The listing builds one solid part. Answer for the finished solid, in the listing's coordinates (mm). Face numbers are marked on the shaded views. A direction names the side the tool comes from. Give positions to 0.01 mm unless a question says otherwise; leave off trailing zeros. Order: outer loops, then holes, each group sorted by start corner. A loop starts at its lowest first (then second) coordinate and runs counter-clockwise, first axis right, second up.
```python
from build123d import *

# Parameters (mm, degrees)
F0_W     = 36
F0_H     = 12
F0_R     = 1.3
F1_DEPTH = 5
F0_W_2   = 12
F0_H_2   = 5
F0_H_3   = 1
F0_H_4   = 2
F2_DEPTH = 2
F3_DEPTH = 8
F4_R     = 2


with BuildPart() as f1:
    # F0 (on Top) → F1 (new body)
    with BuildSketch(Plane.XY):
        with Locations((0, -11)):
            Rectangle(F0_W, F0_H)
        with Locations((-15.25, -14.5)):
            Circle(F0_R, mode=Mode.SUBTRACT)
        with Locations((15.25, -14.5)):
            Circle(F0_R, mode=Mode.SUBTRACT)
    extrude(amount=F1_DEPTH)



with BuildPart() as f1b:
    # F0 (on Top) → F1, piece 2 (new body)
    with BuildSketch(Plane.XY):
        with Locations((-12, 14.5)):
            Rectangle(F0_W_2, F0_H_2)
        with Locations((-15.25, 14.5)):
            Circle(F0_R, mode=Mode.SUBTRACT)
    extrude(amount=F1_DEPTH)


with BuildPart() as f1c:
    # F0 (on Top) → F1, piece 3 (new body)
    with BuildSketch(Plane.XY):
        with Locations((12, 14.5)):
            Rectangle(F0_W_2, F0_H_2)
        with Locations((15.25, 14.5)):
            Circle(F0_R, mode=Mode.SUBTRACT)
    extrude(amount=F1_DEPTH)


with BuildPart() as f1_1:
    add(f1.part)

    add(f1b.part)  # F2 merges F1b

    add(f1c.part)  # F2 merges F1c
    # F0 (on Top) → F2 (join)
    with BuildSketch(Plane.XY):
        Polygon((-6, 12), (-18, 12), (-18, -5), (18, -5), (18, 12), (6, 12), align=None)
        with Locations((0, 14.5)):
            Rectangle(F0_W_2, F0_H_2)
        Polygon((-18, 12), (-18, 17), (-6, 17), (-6, 18), (-19, 18), (-19, -18), (19, -18), (19, 18), (6, 18), (6, 17), (18, 17), (18, 12), (18, -5), (18, -17), (-18, -17), (-18, -5), align=None)
        with Locations((0, 17.5)):
            Rectangle(F0_W_2, F0_H_3)
        with Locations((0, 19)):
            Rectangle(F0_W_2, F0_H_4)
    extrude(amount=F2_DEPTH)

    # F0 (on Top) → F3 (join)
    with BuildSketch(Plane.XY):
        with Locations((-15.25, 14.5)):
            Circle(F0_R)
        with Locations((15.25, 14.5)):
            Circle(F0_R)
        with Locations((15.25, -14.5)):
            Circle(F0_R)
        with Locations((-15.25, -14.5)):
            Circle(F0_R)
        Polygon((-19, 18), (-6, 18), (-6, 20), (-21, 20), (-21, -20), (21, -20), (21, 20), (6, 20), (6, 18), (19, 18), (19, -18), (-19, -18), align=None)
    extrude(amount=F3_DEPTH)

    # F4
    f4_edges = [f1_1.edges().sort_by_distance(p)[0] for p in [
        (-21, -20, 4),
        (21, -20, 4),
        (21, 20, 4),
        (-21, 20, 4),
    ]]
    fillet(f4_edges, radius=F4_R)


solid = f1_1.part
```
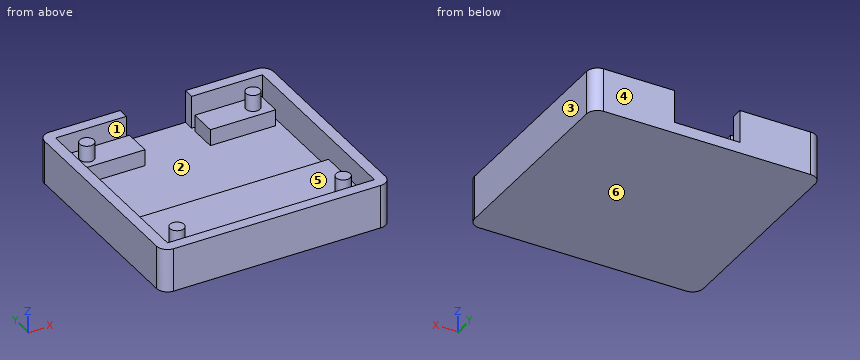
1) For a pull along X with two mould halves and no side action, classify the marked faces 1, 2, 3 and 4 as +X half, -X half, draft (parallel to the pull), parting line (faces both ways), or undercut.
Geometry says:
face 1: undercut
face 2: undercut
face 3: +X half
face 4: draft
2) Find section C-C (x = -3.5). Write down the section's boundary in (y, z).
Geometry says:
outline: (-20, 0) - (20, 0) - (20, 2) - (-5, 2) - (-5, 5) - (-17, 5) - (-17, 2) - (-18, 2) - (-18, 8) - (-20, 8) - close
3) Straight lines are drawn through the part: probe 1 along Y at (x, z) = (15, 4); probe 2 along X at (y, z) = (6.5, 3.5); probe 3 along X at (y, z) = (-10, 4.25). For each, find the intervals that lie inside material, in ascending order.
Geometry says:
probe 1: y = -20 to -18, -17 to -5, 12 to 17, 18 to 20
probe 2: x = -21 to -19, 19 to 21
probe 3: x = -21 to -19, -18 to 18, 19 to 21
4) Find section A-A (z = 3.25). Write down the section's boundary in (x, y), then the cut area to 3 significant figures.
Geometry says:
outline: (-21, -18) arc R2 ccw to (-19, -20) - (19, -20) arc R2 ccw to (21, -18) - (21, 18) arc R2 ccw to (19, 20) - (6, 20) - (6, 18) - (19, 18) - (19, -18) - (-19, -18) - (-19, 18) - (-6, 18) - (-6, 20) - (-19, 20) arc R2 ccw to (-21, 18) - close; (-18, -17) - (18, -17) - (18, -5) - (-18, -5) - close; (-18, 12) - (-6, 12) - (-6, 17) - (-18, 17) - close; (6, 12) - (18, 12) - (18, 17) - (6, 17) - close
area: 837 mm2
5) Find section B-B (y = 16.5). Write down the section's boundary in (x, z).
Geometry says:
outline: (-21, 0) - (21, 0) - (21, 8) - (19, 8) - (19, 2) - (18, 2) - (18, 5) - (6, 5) - (6, 2) - (-6, 2) - (-6, 5) - (-18, 5) - (-18, 2) - (-19, 2) - (-19, 8) - (-21, 8) - close
6) Find section D-D (z = 7.5). Write down the section's boundary in (x, y).
Geometry says:
outline: (-21, -18) arc R2 ccw to (-19, -20) - (19, -20) arc R2 ccw to (21, -18) - (21, 18) arc R2 ccw to (19, 20) - (6, 20) - (6, 18) - (19, 18) - (19, -18) - (-19, -18) - (-19, 18) - (-6, 18) - (-6, 20) - (-19, 20) arc R2 ccw to (-21, 18) - close; circle Ø2.6 at (-15.25, -14.5); circle Ø2.6 at (-15.25, 14.5); circle Ø2.6 at (15.25, -14.5); circle Ø2.6 at (15.25, 14.5)
7) A tool of negligible diameter and unlimited length cuts with its end or side. For the marked faces 5 and 6, from which of +Z, -Z, +X, -X, +Y, -Y can it reach the whole face along a straight path? Write none if from no direction.
Geometry says:
face 5: +Z
face 6: -Z, +X, -X, +Y, -Y
8) Given P1, Ø11.5, axis at x = -9.5, y = -5, coming from the +Z side, flat-ended and moving along its own axis, determine where the tip first touches the part or whether it passes through.
Geometry says:
P1: stops at z = 5
